Check sheet for the drawn part. Datum: minimum x, y, z corner. Units: mm. A direction names the side the tool comes from. Give positions to 0.01 mm unless a question says otherwise; leave off trailing zeros. Write each loop counter-clockwise with the first axis right and the second up, starting at its lowest first coordinate (ties: lowest second). Pieces come first, ordered by that corner, then holes. Notation, with made-up numbers: (33, -23.75) - (53, -23.75) arc R25 cw to (53, 10.25) - close; hole circle Ø10 at (-30, 65.25). An arc over 180 degrees is marked (long way). Return JSON: item names as keys, results as strings. Group by question number.
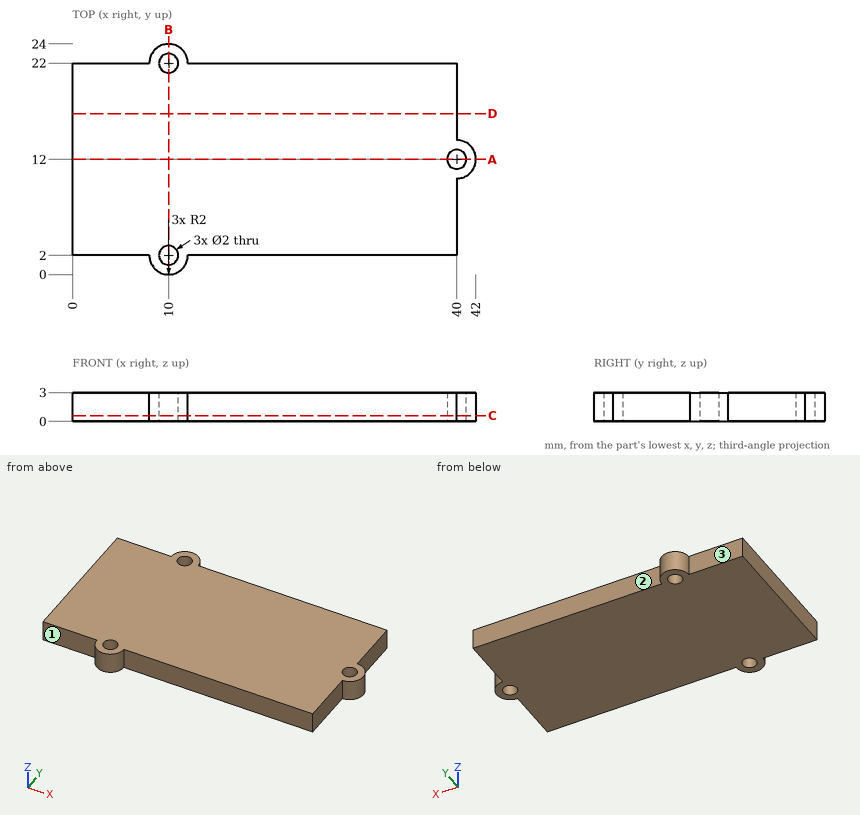
Item 1: Section check A-A on y = 12. Record the cut outline in (x, z).
Item 2: Material ranges on line 1 along Y through (x, z) = (10, 1.7); line 2 along X through (y, z) = (4, 2.75); line 3 along Y through (x, z) = (23.5, 0.4), recorded low to high. Write a range as from..to.
Item 3: Depth check by flat-ended pin: pin 1 (5 mm diameter, centred on x = 28.5, y = 6, fed in from -Z); pin 2 (1.5 mm diameter, centred on y = 6.5, z = 2, fed in from +X); pin 3 (1.5 mm diameter, centred on x = 18.5, z = 1, fed in from -Y); pin 4 (1.5 mm diameter, centred on x = 31.5, z = 2, fed in from +Y). Enter the tip coordinate at first touch or a pass-through.
Item 4: Section check B-B on x = 10. Record the cut outline in (y, z).
Item 5: Access from +Z, -Z, +X, -X, +Y, -Y to the whole of each face (thin tool, end or side, straight path). Record for the marked faces 1, 2 and 3.
Item 6: Section check C-C on z = 0.6. Record the cut outline in (x, y).
Item 7: Section check D-D on y = 16.75. Record the cut outline in (x, z), plus the area to 3 significant figures.
Reply:
{
 "1": {"outline": "(0, 0) - (39, 0) - (39, 3) - (0, 3) - close; (41, 0) - (42, 0) - (42, 3) - (41, 3) - close"},
 "2": {"line 1": "0..1, 3..21, 23..24", "line 2": "0..40", "line 3": "2..22"},
 "3": {"pin 1": "z = 0", "pin 2": "x = 40", "pin 3": "y = 2", "pin 4": "y = 22"},
 "4": {"outline": "(0, 0) - (1, 0) - (1, 3) - (0, 3) - close; (3, 0) - (21, 0) - (21, 3) - (3, 3) - close; (23, 0) - (24, 0) - (24, 3) - (23, 3) - close"},
 "5": {"face 1": "+Z, -Z, -X, -Y", "face 2": "+Z, -Z, +X, +Y", "face 3": "+Z, -Z, -X, +Y"},
 "6": {"outline": "(0, 2) - (8, 2) arc R2 ccw to (12, 2) - (40, 2) - (40, 10) arc R2 ccw to (40, 14) - (40, 22) - (12, 22) arc R2 ccw to (8, 22) - (0, 22) - close; hole circle Ø2 at (10, 2); hole circle Ø2 at (10, 22); hole circle Ø2 at (40, 12)"},
 "7": {"outline": "(0, 0) - (40, 0) - (40, 3) - (0, 3) - close", "area": "120 mm²"}
}
